The listing builds one solid part. Answer for the finished solid, in the listing's coordinates (mm). Give positions to 0.01 mm unless a question says otherwise; leave off trailing zeros. Order: outer loops, then holes, each group sorted by start corner. A loop starts at its lowest first (then second) coordinate and runs counter-clockwise, first axis right, second up. Notation, with made-up numbers: (3.25, 85) - (44.25, 85) arc R19 cw to (44.25, 105) - close; hole circle Ø3 at (48.5, 72). An arc over 180 degrees is marked (long way). Answer as CSV lines item,"result". Start each with the question number.
1. Section D-D on x = 1.5 is taken. Give the vertices of the cut face in (y, z).
2. Section C-C on z = 2.5 is taken. Give the vertices of the cut face in (x, y).
3. Consider line 1 along Y through (x, z) = (110, 3.8); line 2 along X through (y, z) = (-1.25, 0.75); line 3 along Z through (x, y) = (20, 6.5). Determine where each line is inside the solid, lowest interval first. Write a range as [from, to].
4. Flat-ended cylindrical pins translate along their axes: pin 1 (1 mm diameter, centred on y = -3.5, z = 3, fed in from +X); pin 2 (10 mm diameter, centred on x = 46, y = 0.5, fed in from -Z); pin 3 (5 mm diameter, centred on x = 1.5, y = 2, fed in from -Z). Find the tip coordinate at first contact, or state that the pin passes through.
5. Section B-B on x = 20 is taken. Give the vertices of the cut face in (y, z), and give its area (3 significant figures).
6. Section A-A on y = 0 is taken. Give the vertices of the cut face in (x, z), and give its area (3 significant figures).
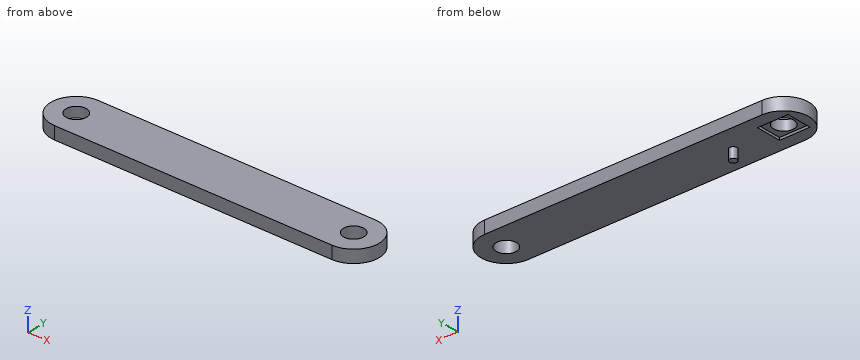
from build123d import *

# Parameters (mm, degrees)
SKETCH1_R           = 4.01
BOSS_EXTRUDE1_DEPTH = 5
SKETCH2_R           = 1.49
BOSS_EXTRUDE3_DEPTH = 4
SKETCH5_W           = 12.1
SKETCH5_H           = 10.1
CUT_EXTRUDE1_DEPTH  = 1


with BuildPart() as part:
    # Sketch1 → Boss-Extrude1 (new body)
    with BuildSketch(Plane.XY):
        with BuildLine():
            Line((110, 10), (0, 10))
            ThreePointArc((0, 10), (-10, 0), (0, -10))
            Line((0, -10), (110, -10))
            ThreePointArc((110, -10), (120, 0), (110, 10))
        make_face()
        Circle(SKETCH1_R, mode=Mode.SUBTRACT)
        with Locations((110, 0)):
            Circle(SKETCH1_R, mode=Mode.SUBTRACT)
    extrude(amount=BOSS_EXTRUDE1_DEPTH)

    # Sketch2 → Boss-Extrude3 (add)
    with BuildSketch(Plane(origin=(0, 0, 0), x_dir=(-1, 0, 0), z_dir=(0, 0, -1))):
        with Locations(Location((-20, 0, 0), (0, 0, 180))):
            Circle(SKETCH2_R)
    extrude(amount=BOSS_EXTRUDE3_DEPTH)

    # Sketch5 → Cut-Extrude1 (cut)
    with BuildSketch(Plane(origin=(0, 0, 0), x_dir=(-1, 0, 0), z_dir=(0, 0, -1))):
        Rectangle(SKETCH5_W, SKETCH5_H)
    extrude(amount=-CUT_EXTRUDE1_DEPTH, mode=Mode.SUBTRACT)


solid = part.part
Checks:
1,outline,"(-10, 0) - (-5.05, 0) - (-5.05, 1) - (-3.72, 1) - (-3.72, 5) - (-10, 5) - close; (3.72, 1) - (5.05, 1) - (5.05, 0) - (10, 0) - (10, 5) - (3.72, 5) - close"
2,outline,"(0, -10) - (110, -10) arc R10 ccw to (110, 10) - (0, 10) arc R10 ccw to start; hole circle Ø8.02 at (0, 0); hole circle Ø8.02 at (110, 0)"
3,line 1,"y = [-10, -4.01], [4.01, 10]"
3,line 2,"x = [-9.92, -6.05], [6.05, 106.19], [113.81, 119.92]"
3,line 3,"z = [0, 5]"
4,pin 1,"stops at x = 119.54"
4,pin 2,"stops at z = 0"
4,pin 3,"stops at z = 1"
5,outline,"(-10, 0) - (-1.49, 0) - (-1.49, -4) - (1.49, -4) - (1.49, 0) - (10, 0) - (10, 5) - (-10, 5) - close"
5,area,"112 mm²"
6,outline,"(-10, 0) - (-6.05, 0) - (-6.05, 1) - (-4.01, 1) - (-4.01, 5) - (-10, 5) - close; (4.01, 1) - (6.05, 1) - (6.05, 0) - (18.51, 0) - (18.51, -4) - (21.49, -4) - (21.49, 0) - (105.99, 0) - (105.99, 5) - (4.01, 5) - close; (114.01, 0) - (120, 0) - (120, 5) - (114.01, 5) - close"
6,area,"578 mm²"
